The listing builds one solid part. Answer for the finished solid, in the listing's coordinates (mm). A direction names the side the tool comes from. Coordinates: 2 decimals unless noted, no trailing zeros. Order: outer loops, then holes, each group sorted by start corner. A loop starts at its lowest first (then second) coordinate and runs counter-clockwise, first axis right, second up. Notation, with made-up numbers: (26.25, -30.5) - (34.25, -30.5) arc R24 ccw to (34.25, -14.5) - close; hole circle Ø11 at (-13.75, 75). An arc over 180 degrees is marked (long way). Use one line per item in the form item = value. Start each with the question number.
Item 1: Section C-C, the plane x = 74 is taken. Write down the section's boundary in (y, z).
Item 2: The mould has two halves that part along X. Classify faces 1 (the flat face through (86.75, 5, -55)), 2 (the flat face through (-30.25, 5, -10)), 3 (the flat face through (27.25, 9, 1)), 4 (the flat face through (79, 3, -48)): released by +X, released by -X, zero draft, split by the parting line, or undercut.
Item 3: Section D-D, the plane x = 3 is taken. Write down the section's boundary in (y, z), and give its area (3 significant figures).
Item 4: A tool of negligible diameter and unlimited length cuts with its end or side. For faces 5 (the flat face through (-27.25, 7, 1)), 6 (the flat face through (55, 3, -75)), 7 (the flat face through (48, 3, -85)), from which of +Z, -Z, +X, -X, +Y, -Y can it reach the whole face along a straight path? Write none if from no direction.
Item 5: Consider line 1 along X through (y, z) = (3.6, -48); line 2 along X through (y, z) = (1.95, -75); line 3 along X through (y, z) = (7.75, -56.5). Determine where each line is inside the solid, lowest interval first. Write a range as [from, to].
Item 6: Each of these flat-tipped pins is pushed along its axis until it touches: pin 1 Ø12 at (x, z) = (58, -72.5) entering from +Y; pin 2 Ø6.5 at (y, z) = (6, 27.5) entering from +X; pin 3 Ø3.5 at (x, z) = (29.5, -68) entering from -Y. Where does it stop, or does it pass through?
Item 7: Section B-B, the plane z = -6.5 is taken. Write down the section's boundary in (x, y).
Item 8: Section A-A, the plane x = -20.25 is taken. Write down the section's boundary in (y, z).
from build123d import *

# Parameters (mm, degrees)
SKETCH1_W               = 60.5
SKETCH1_H               = 170
BOSS_EXTRUDE1_DEPTH     = 11
SKETCH2_W               = 54.5
SKETCH2_H               = 167
CUT_EXTRUDE1_DEPTH      = 8
SKETCH3_W               = 12
SKETCH3_H               = 3
CUT_EXTRUDE2_DEPTH      = 8
SKETCH4_W               = 20
SKETCH4_H               = 20
SKETCH4_R               = 2.75
BOSS_EXTRUDE3_DEPTH     = 3
SKETCH5_W               = 5
SKETCH5_H               = 5.5
CUT_EXTRUDE3_DEPTH      = 16
SKETCH7_W               = 56.5
SKETCH7_H               = 60
SKETCH7_R               = 1.75
BOSS_EXTRUDE7_DEPTH     = 3
SKETCH9_W               = 38.3
SKETCH9_H               = 16.65
SKETCH9_W_2             = 30
SKETCH9_H_2             = 5
BOSS_EXTRUDE8_DEPTH     = 1.4
SKETCH10_W              = 3
SKETCH10_H              = 60
BOSS_EXTRUDE9_DEPTH     = 6
SKETCH12_R              = 2.75
CUT_EXTRUDE4_DEPTH      = 3
SKETCH13_W              = 20.5
SKETCH13_H              = 5
SKETCH13_W_2            = 30
SKETCH13_W_3            = 5
SKETCH13_H_2            = 172
BOSS_EXTRUDE10_DEPTH    = 2
SKETCH14_W              = 38.3
SKETCH14_H              = 16.65
SKETCH14_W_2            = 30
SKETCH14_H_2            = 5
BOSS_EXTRUDE11_DEPTH    = 3
SKETCH15_W              = 53.5
SKETCH15_H              = 60
SKETCH15_R              = 1.75
SKETCH15_R_2            = 2.75
BOSS_EXTRUDE12_DEPTH    = 3
SKETCH16_R              = 1.75
CUT_EXTRUDE5_DEPTH      = 3
CUT_EXTRUDE6_START      = -3
SKETCH17_R              = 7.5
SKETCH17_R_2            = 2.75
CUT_EXTRUDE6_DEPTH      = 3
SKETCH18_W              = 20
SKETCH18_H              = 3
CUT_EXTRUDE7_DEPTH      = 3
CUT_EXTRUDE8_DEPTH      = 135.140085359
CUT_EXTRUDE8_DEPTH_BACK = 135.140085359
SKETCH19_W              = 25
SKETCH19_H              = 130


with BuildPart() as part:
    # Sketch1 → Boss-Extrude1 (new body)
    with BuildSketch(Plane(origin=(0, 0, 0), x_dir=(1, 0, 0), z_dir=(0, 1, 0))):
        Rectangle(SKETCH1_W, SKETCH1_H)
    extrude(amount=BOSS_EXTRUDE1_DEPTH)

    # Sketch2 → Cut-Extrude1 (cut)
    with BuildSketch(Plane(origin=(0, 11, 0), x_dir=(1, 0, 0), z_dir=(0, 1, 0))):
        with Locations((0, 1.5)):
            Rectangle(SKETCH2_W, SKETCH2_H)
    extrude(amount=-CUT_EXTRUDE1_DEPTH, mode=Mode.SUBTRACT)

    # Sketch3 → Cut-Extrude2 (cut)
    with BuildSketch(Plane(origin=(0, 11, 0), x_dir=(1, 0, 0), z_dir=(0, 1, 0))):
        with Locations((-21.25, -83.5)):
            Rectangle(SKETCH3_W, SKETCH3_H)
        with Locations((21.25, -83.5)):
            Rectangle(SKETCH3_W, SKETCH3_H)
    extrude(amount=-CUT_EXTRUDE2_DEPTH, mode=Mode.SUBTRACT)

    # Sketch4 → Boss-Extrude3 (add)
    with BuildSketch(Plane.XZ):
        with Locations((-20.25, -95)):
            Rectangle(SKETCH4_W, SKETCH4_H)
        with Locations(Location((-20.25, -95, 0), (0, 0, 270))):
            Circle(SKETCH4_R, mode=Mode.SUBTRACT)
    extrude(amount=-BOSS_EXTRUDE3_DEPTH)

    # Sketch5 → Cut-Extrude3 (cut)
    with BuildSketch(Plane.ZY.offset(-27.25)):
        with Locations((66.5, 5.75)):
            Rectangle(SKETCH5_W, SKETCH5_H)
        with Locations((-0.5, 5.75)):
            Rectangle(SKETCH5_W, SKETCH5_H)
        with Locations((-67.5, 5.75)):
            Rectangle(SKETCH5_W, SKETCH5_H)
    extrude(amount=-CUT_EXTRUDE3_DEPTH, mode=Mode.SUBTRACT)

    # Sketch7 → Boss-Extrude7 (add)
    with BuildSketch(Plane.XZ):
        with Locations((58.5, -55)):
            Rectangle(SKETCH7_W, SKETCH7_H)
        with Locations(Location((81.25, -48, 0), (0, 0, 270))):
            Circle(SKETCH7_R, mode=Mode.SUBTRACT)
        with Locations(Location((32.95, -41.65, 0), (0, 0, 270))):
            Circle(SKETCH7_R, mode=Mode.SUBTRACT)
    extrude(amount=-BOSS_EXTRUDE7_DEPTH)

    # Sketch9 → Boss-Extrude8 (add)
    with BuildSketch(Plane(origin=(0, 3, 0), x_dir=(1, 0, 0), z_dir=(0, 1, 0))):
        with Locations((57.1, 33.325)):
            Rectangle(SKETCH9_W, SKETCH9_H)
        with Locations((63.25, 52)):
            Rectangle(SKETCH9_W_2, SKETCH9_H_2)
    extrude(amount=BOSS_EXTRUDE8_DEPTH)

    # Sketch10 → Boss-Extrude9 (add)
    with BuildSketch(Plane(origin=(0, 3, 0), x_dir=(1, 0, 0), z_dir=(0, 1, 0))):
        with Locations((85.25, 55)):
            Rectangle(SKETCH10_W, SKETCH10_H)
    extrude(amount=BOSS_EXTRUDE9_DEPTH)

    # Sketch12 → Cut-Extrude4 (cut)
    with BuildSketch(Plane(origin=(0, 3, 0), x_dir=(1, 0, 0), z_dir=(0, 1, 0))):
        with Locations(Location((58.25, 75, 0), (0, 0, 270))):
            Circle(SKETCH12_R)
    extrude(amount=-CUT_EXTRUDE4_DEPTH, mode=Mode.SUBTRACT)

    # Sketch13 → Boss-Extrude10 (add)
    with BuildSketch(Plane.XZ):
        with Locations((76.5, -75)):
            Rectangle(SKETCH13_W, SKETCH13_H)
        with Locations((35.25, -75)):
            Rectangle(SKETCH13_W_2, SKETCH13_H)
        with Locations((-20.25, -1)):
            Rectangle(SKETCH13_W_3, SKETCH13_H_2)
    extrude(amount=BOSS_EXTRUDE10_DEPTH)

    # Sketch14 → Boss-Extrude11 (add)
    with BuildSketch(Plane(origin=(0, 4.4, 0), x_dir=(1, 0, 0), z_dir=(0, 1, 0))):
        with Locations((57.1, 33.325)):
            Rectangle(SKETCH14_W, SKETCH14_H)
        with Locations((63.25, 52)):
            Rectangle(SKETCH14_W_2, SKETCH14_H_2)
    extrude(amount=BOSS_EXTRUDE11_DEPTH)

    # Sketch15 → Boss-Extrude12 (add)
    with BuildSketch(Plane(origin=(0, 3, 0), x_dir=(1, 0, 0), z_dir=(0, 1, 0))):
        with Locations((57, 55)):
            Rectangle(SKETCH15_W, SKETCH15_H)
        with Locations(Location((32.95, 41.65, 0), (0, 0, 90))):
            Circle(SKETCH15_R, mode=Mode.SUBTRACT)
        with Locations(Location((81.25, 48, 0), (0, 0, 90))):
            Circle(SKETCH15_R, mode=Mode.SUBTRACT)
        with Locations(Location((58.25, 75, 0), (0, 0, 270))):
            Circle(SKETCH15_R_2, mode=Mode.SUBTRACT)
    extrude(amount=BOSS_EXTRUDE12_DEPTH)

    # Sketch16 → Cut-Extrude5 (cut)
    # profile 1 of 2: a face of its own
    with BuildSketch(Plane.XZ):
        Polygon((81.25, -44.824573519), (78.5, -46.41228676), (78.5, -49.58771324), (81.25, -51.175426481), (84, -49.58771324), (84, -46.41228676), align=None)
        with Locations(Location((81.25, -48, 0), (0, 0, 270))):
            Circle(SKETCH16_R, mode=Mode.SUBTRACT)
    # profile 2 of 2: a face of its own
    with BuildSketch(Plane.XZ):
        Polygon((32.95, -38.474573519), (30.2, -40.06228676), (30.2, -43.23771324), (32.95, -44.825426481), (35.7, -43.23771324), (35.7, -40.06228676), align=None)
        with Locations(Location((32.95, -41.65, 0), (0, 0, 270))):
            Circle(SKETCH16_R, mode=Mode.SUBTRACT)
    extrude(amount=-CUT_EXTRUDE5_DEPTH, mode=Mode.SUBTRACT)

    # Sketch17 → Cut-Extrude6 (cut)
    with BuildSketch(Plane(origin=(0, 6, 0), x_dir=(1, 0, 0), z_dir=(0, 1, 0)).offset(CUT_EXTRUDE6_START)):
        with Locations(Location((58.25, 75, 0), (0, 0, 270))):
            Circle(SKETCH17_R)
        with Locations(Location((58.25, 75, 0), (0, 0, 270))):
            Circle(SKETCH17_R_2, mode=Mode.SUBTRACT)
    extrude(amount=CUT_EXTRUDE6_DEPTH, mode=Mode.SUBTRACT)

    # Sketch18 → Cut-Extrude7 (cut)
    with BuildSketch(Plane(origin=(0, 0, -105), x_dir=(-1, 0, 0), z_dir=(0, 0, -1))):
        with Locations((20.25, 1.5)):
            Rectangle(SKETCH18_W, SKETCH18_H)
    extrude(amount=-CUT_EXTRUDE7_DEPTH, mode=Mode.SUBTRACT)

    # Sketch19 → Cut-Extrude8 (cut, two sides: drawn at the far end of the back side and taken through both)
    with BuildSketch(Plane(origin=(0, 3, 0), x_dir=(1, 0, 0), z_dir=(0, 1, 0)).offset(-CUT_EXTRUDE8_DEPTH_BACK)):
        Rectangle(SKETCH19_W, SKETCH19_H)
    extrude(amount=CUT_EXTRUDE8_DEPTH + CUT_EXTRUDE8_DEPTH_BACK, mode=Mode.SUBTRACT)


solid = part.part
Response:
q1.outline = (-2, -77.5) - (0, -77.5) - (0, -85) - (6, -85) - (6, -54.5) - (7.4, -54.5) - (7.4, -49.5) - (6, -49.5) - (6, -41.65) - (7.4, -41.65) - (7.4, -25) - (0, -25) - (0, -72.5) - (-2, -72.5) - close
q2.face_1 = released by +X
q2.face_2 = released by -X
q2.face_3 = undercut
q2.face_4 = undercut
q3.outline = (0, -85) - (3, -85) - (3, -65) - (0, -65) - close; (0, 65) - (3, 65) - (3, 82) - (11, 82) - (11, 85) - (0, 85) - close
q3.area = 144 mm2
q4.face_5 = +Z, -Z, +Y
q4.face_6 = +Y
q4.face_7 = -Z, +X, +Y, -Y
q5.line_1 = [-30.25, -27.25], [27.25, 79.5], [83, 86.75]
q5.line_2 = [-30.25, 55.5], [61, 86.75]
q5.line_3 = [-30.25, -27.25], [27.25, 30.25], [83.75, 86.75]
q6.pin_1 = 6
q6.pin_2 = 30.25
q6.pin_3 = 0
q7.outline = (-30.25, 0) - (-22.75, 0) - (-22.75, -2) - (-17.75, -2) - (-17.75, 0) - (-12.5, 0) - (-12.5, 3) - (-27.25, 3) - (-27.25, 11) - (-30.25, 11) - close; (12.5, 0) - (30.25, 0) - (30.25, 11) - (27.25, 11) - (27.25, 3) - (12.5, 3) - close
q8.outline = (-2, -87) - (0, -87) - (0, -92.25) - (3, -92.25) - (3, 85) - (-2, 85) - close; (0, -102) - (3, -102) - (3, -97.75) - (0, -97.75) - close
